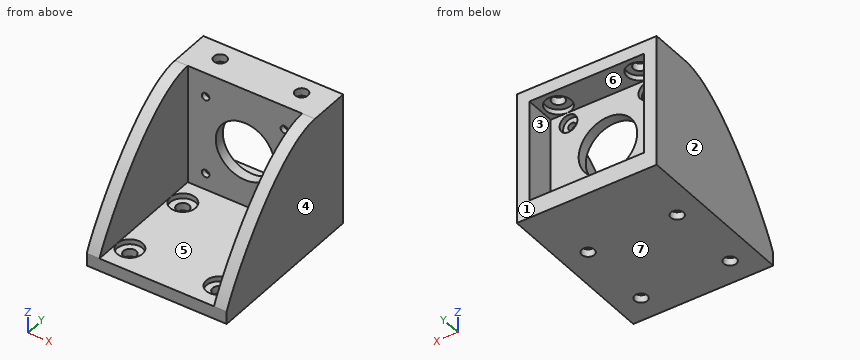
from build123d import *

# Parameters (mm, degrees)
SKETCH1_W           = 55
SKETCH1_H           = 50
SKETCH1_R           = 2.5
BOSS_EXTRUDE1_DEPTH = 5
SKETCH2_R           = 5
CUT_EXTRUDE1_DEPTH  = 2
SKETCH3_W           = 55
SKETCH3_H           = 52
BOSS_EXTRUDE2_DEPTH = 16
SKETCH4_R           = 11.5
SKETCH4_R_2         = 1.5
CUT_EXTRUDE2_DEPTH  = 17
BOSS_EXTRUDE3_DEPTH = 5
SKETCH6_W           = 45
SKETCH6_H           = 40
CUT_EXTRUDE3_DEPTH  = 12
SKETCH7_R           = 3.5
CUT_EXTRUDE4_DEPTH  = 2
SKETCH8_R           = 2.5
CUT_EXTRUDE5_DEPTH  = 5
SKETCH10_R          = 5
CUT_EXTRUDE6_DEPTH  = 2


with BuildPart() as part:
    # Sketch1 → Boss-Extrude1 (new body)
    with BuildSketch(Plane.XY):
        Rectangle(SKETCH1_W, SKETCH1_H)
        with Locations((-17.5, -15)):
            Circle(SKETCH1_R, mode=Mode.SUBTRACT)
        with Locations((17.5, -15)):
            Circle(SKETCH1_R, mode=Mode.SUBTRACT)
        with Locations((-17.5, 15)):
            Circle(SKETCH1_R, mode=Mode.SUBTRACT)
        with Locations((17.5, 15)):
            Circle(SKETCH1_R, mode=Mode.SUBTRACT)
    extrude(amount=BOSS_EXTRUDE1_DEPTH)

    # Sketch2 → Cut-Extrude1 (cut)
    with BuildSketch(Plane.XY.offset(5)):
        with Locations((-17.5, -15)):
            Circle(SKETCH2_R)
        with Locations((17.5, -15)):
            Circle(SKETCH2_R)
        with Locations((-17.5, 15)):
            Circle(SKETCH2_R)
        with Locations((17.5, 15)):
            Circle(SKETCH2_R)
    extrude(amount=-CUT_EXTRUDE1_DEPTH, mode=Mode.SUBTRACT)

    # Sketch3 → Boss-Extrude2 (add)
    with BuildSketch(Plane(origin=(0, 25, 0), x_dir=(1, 0, 0), z_dir=(0, 1, 0))):
        with Locations((0, -26)):
            Rectangle(SKETCH3_W, SKETCH3_H)
    extrude(amount=BOSS_EXTRUDE2_DEPTH)

    # Sketch4 → Cut-Extrude2 (cut, through all)
    with BuildSketch(Plane(origin=(0, 25, 0), x_dir=(-1, 0, 0), z_dir=(0, -1, 0))):
        with Locations((0, -27)):
            Circle(SKETCH4_R)
        with Locations((15.5, -42.5)):
            Circle(SKETCH4_R_2)
        with Locations((-15.5, -42.5)):
            Circle(SKETCH4_R_2)
        with Locations((-15.5, -11.5)):
            Circle(SKETCH4_R_2)
        with Locations((15.5, -11.5)):
            Circle(SKETCH4_R_2)
    extrude(amount=-CUT_EXTRUDE2_DEPTH, mode=Mode.SUBTRACT)

    # Sketch5 → Boss-Extrude3 (add)
    with BuildSketch(Plane.ZY.offset(27.5)):
        with BuildLine():
            Line((5, -25), (5, 25))
            Line((5, 25), (52, 25))
            add(Edge.make_bspline(
                [(52, 25), (52, 4.232970162), (15.26663468, -20.719918254), (5, -25)],
                knots=[0, 0, 0, 0, 0.911487557, 0.911487557, 0.911487557, 0.911487557], degree=3))
        make_face()
    boss_extrude3 = extrude(amount=-BOSS_EXTRUDE3_DEPTH)

    # Mirror1: Boss-Extrude3 across plane
    add(boss_extrude3.mirror(Plane(origin=(0, 0, 0), x_dir=(0, 0, 1), z_dir=(1, 0, 0))))

    # Sketch6 → Cut-Extrude3 (cut)
    with BuildSketch(Plane(origin=(0, 41, 0), x_dir=(1, 0, 0), z_dir=(0, 1, 0))):
        with Locations((0, -27)):
            Rectangle(SKETCH6_W, SKETCH6_H)
    extrude(amount=-CUT_EXTRUDE3_DEPTH, mode=Mode.SUBTRACT)

    # Sketch7 → Cut-Extrude4 (cut)
    with BuildSketch(Plane(origin=(0, 29, 0), x_dir=(1, 0, 0), z_dir=(0, 1, 0))):
        with Locations((-15.5, -11.5)):
            Circle(SKETCH7_R)
        with Locations((15.5, -11.5)):
            Circle(SKETCH7_R)
        with Locations((15.5, -42.5)):
            Circle(SKETCH7_R)
        with Locations((-15.5, -42.5)):
            Circle(SKETCH7_R)
    extrude(amount=-CUT_EXTRUDE4_DEPTH, mode=Mode.SUBTRACT)

    # Sketch8 → Cut-Extrude5 (cut)
    with BuildSketch(Plane.XY.offset(52)):
        with Locations((16, 34)):
            Circle(SKETCH8_R)
        with Locations((-16, 34)):
            Circle(SKETCH8_R)
    extrude(amount=-CUT_EXTRUDE5_DEPTH, mode=Mode.SUBTRACT)

    # Sketch10 → Cut-Extrude6 (cut)
    with BuildSketch(Plane(origin=(0, 0, 47), x_dir=(-1, 0, 0), z_dir=(0, 0, -1))):
        with Locations((-16, 34)):
            Circle(SKETCH10_R)
        with Locations((16, 34)):
            Circle(SKETCH10_R)
    extrude(amount=-CUT_EXTRUDE6_DEPTH, mode=Mode.SUBTRACT)


solid = part.part
CAD build for the part. Positions are in the model's coordinates, mm. Face numbers are marked on the shaded views. A direction names the side the tool comes from. Give positions to 0.01 mm unless a question says otherwise; leave off trailing zeros. Order: outer loops, then holes, each group sorted by start corner. A loop starts at its lowest first (then second) coordinate and runs counter-clockwise, first axis right, second up. Notation, with made-up numbers: (-11.75, -14.75) - (1.25, -14.75) arc R17 ccw to (1.25, -10.75) - close; hole circle Ø11 at (76, 60.25). An arc over 180 degrees is marked (long way). Write each question's results on one line, items separated by ' | '.
1. Probe L1, parallel to X at y = 26.15, z = 11.5; L2, parallel to Y at x = -17.5, z = 4.55; L3, parallel to X at y = -15, z = 1. List the from-to ranges inside material, lowest first. Write a range as from..to.
Calculated:
L1: x = -27.5..-17, -14..14, 17..27.5 | L2: y = -25..-20, -10..10, 20..41 | L3: x = -27.5..-20, -15..15, 20..27.5
2. Saw through at B-B on x = 0. List the corners of the cut face in (y, z).
Calculated:
outline: (-25, 0) - (41, 0) - (41, 7) - (29, 7) - (29, 15.5) - (25, 15.5) - (25, 5) - (-25, 5) - close; (25, 38.5) - (29, 38.5) - (29, 47) - (41, 47) - (41, 52) - (25, 52) - close
3. Pull direction X, two halves, no side cores. Call the marked faces 1, 2, 3 and 4: released by +X, released by -X, zero draft, split by the parting line, or undercut.
Calculated:
face 1: zero draft | face 2: released by -X | face 3: undercut | face 4: released by +X
4. Saw through at D-D on z = 42.5. Count the separate pieces of the cut face and the enclosed holes in it, and give its area (3 significant figures).
Calculated:
separate pieces: 3 | enclosed holes: 0 | area: 508 mm2
5. 3-axis set-ups, long thin cutter, end or side, ignore diameter. For the marked faces 5, 6 and 7: which of +Z, -Z, +X, -X, +Y, -Y reach the whole face in a straight line?
Calculated:
face 5: +Z, -Y | face 6: +Y | face 7: -Z, +X, -X, +Y, -Y
6. Saw through at A-A on y = 34. List the corners of the cut face in (x, z), and give its area (3 significant figures).
Calculated:
outline: (-27.5, 0) - (27.5, 0) - (27.5, 52) - (18.5, 52) - (18.5, 49) - (21, 49) - (21, 47) - (22.5, 47) - (22.5, 7) - (-22.5, 7) - (-22.5, 47) - (-21, 47) - (-21, 49) - (-18.5, 49) - (-18.5, 52) - (-27.5, 52) - close; (-13.5, 49) - (-11, 49) - (-11, 47) - (11, 47) - (11, 49) - (13.5, 49) - (13.5, 52) - (-13.5, 52) - close | area: 990 mm2
7. Pin check, flat tips, straight feed: pin 1 (10 mm diameter, centred on x = -10, z = 26.5, fed in from -Y); pin 2 (3 mm diameter, centred on x = -17.5, y = 15.5, fed in from +Z); pin 3 (3.5 mm diameter, centred on x = 15.5, z = 11.5, fed in from +Y); pin 4 (8 mm diameter, centred on x = 17.5, y = 15, fed in from +Z). Stop position of each tip, or through.
Calculated:
pin 1: stops at y = 25 | pin 2: passes through | pin 3: stops at y = 27 | pin 4: stops at z = 3
8. Saw through at C-C on x = -9.5. List the corners of the cut face in (y, z).
Calculated:
outline: (-25, 0) - (41, 0) - (41, 7) - (29, 7) - (29, 20.52) - (25, 20.52) - (25, 5) - (-25, 5) - close; (25, 33.48) - (29, 33.48) - (29, 47) - (41, 47) - (41, 52) - (25, 52) - close
